Check sheet for the drawn part. Datum: minimum x, y, z corner. Units: mm. Coordinates: 2 decimals unless noted, no trailing zeros. Order: outer loops, then holes, each group sorted by start corner. A loop starts at its lowest first (then second) coordinate and runs counter-clockwise, first axis right, second up. Notation, with made-up numbers: (-6.75, 2) - (11.25, 2) arc R28 ccw to (11.25, 34) - close; hole circle Ø10 at (88, 0.25). An arc over 180 degrees is marked (long way). Put each result on its own line as item: value.
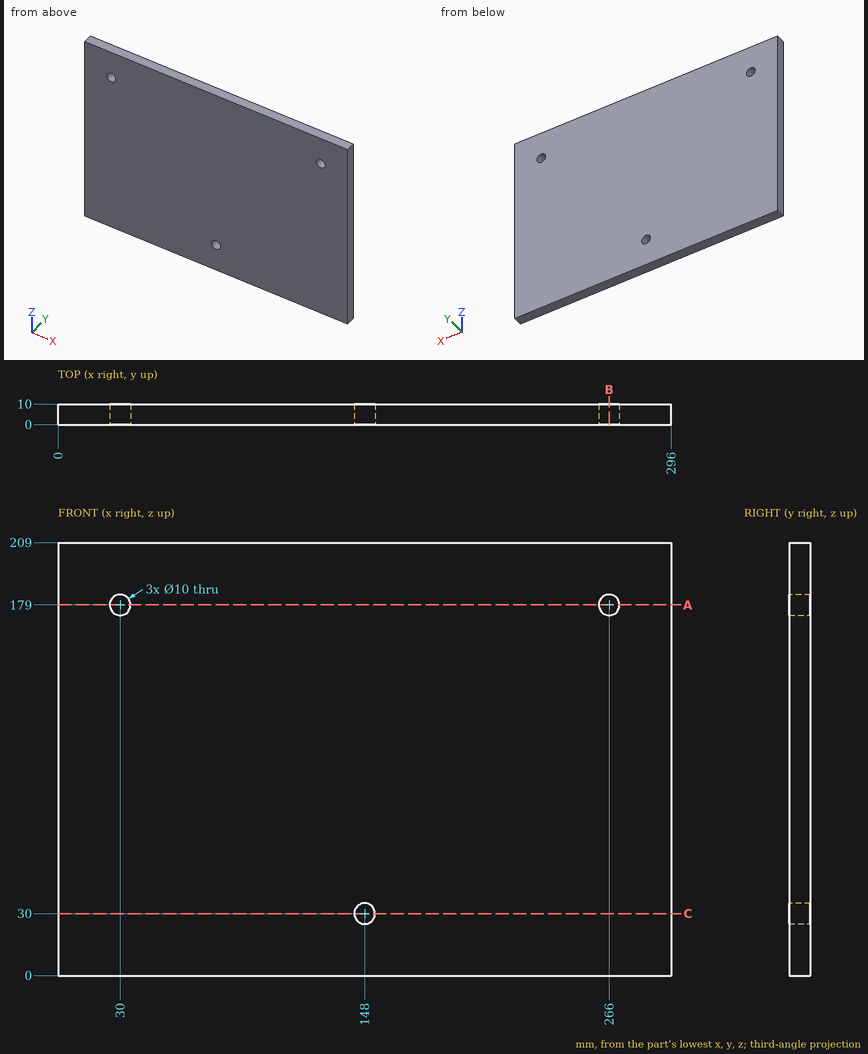
Q1. Section check C-C on z = 30. Record the boundary of the cut face in (x, y).
Answer block:
outline: (0, 0) - (143, 0) - (143, 10) - (0, 10) - close; (153, 0) - (296, 0) - (296, 10) - (153, 10) - close
Q2. Depth check by flat-ended pin: pin 1 Ø6 at (x, z) = (148, 30) entering from +Y. Enter the tip coordinate at first touch or a pass-through.
Answer block:
pin 1: passes through
Q3. Thickness scan on L1, parallel to X at y = 4.75, z = 179; L2, parallel to X at y = 4.5, z = 30; L3, parallel to Z at x = 33, y = 3.75. Record the ranges inside material, lowest first. Write a range as [from, to].
Answer block:
L1: x = [0, 25], [35, 261], [271, 296]
L2: x = [0, 143], [153, 296]
L3: z = [0, 175], [183, 209]
Q4. Section check A-A on z = 179. Record the boundary of the cut face in (x, y).
Answer block:
outline: (0, 0) - (25, 0) - (25, 10) - (0, 10) - close; (35, 0) - (261, 0) - (261, 10) - (35, 10) - close; (271, 0) - (296, 0) - (296, 10) - (271, 10) - close
Q5. Section check B-B on x = 266. Record the boundary of the cut face in (y, z), then the cut area to 3 significant figures.
Answer block:
outline: (0, 0) - (10, 0) - (10, 174) - (0, 174) - close; (0, 184) - (10, 184) - (10, 209) - (0, 209) - close
area: 1,990 mm^2
